from build123d import *

# Parameters (mm, degrees)
SKETCH1_R           = 23.25
BOSS_EXTRUDE1_DEPTH = 8
SKETCH2_R           = 9.6
CUT_EXTRUDE1_DEPTH  = 6.2
SKETCH3_R           = 5
CUT_EXTRUDE2_DEPTH  = 1.8
CHAMFER1_SIZE       = 2


with BuildPart() as part:
    # Sketch1 → Boss-Extrude1 (new body)
    with BuildSketch(Plane.XY):
        Circle(SKETCH1_R)
    extrude(amount=BOSS_EXTRUDE1_DEPTH)

    # Sketch2 → Cut-Extrude1 (cut)
    with BuildSketch(Plane.XY.offset(8)):
        Circle(SKETCH2_R)
    extrude(amount=-CUT_EXTRUDE1_DEPTH, mode=Mode.SUBTRACT)

    # Sketch3 → Cut-Extrude2 (cut)
    with BuildSketch(Plane.XY.offset(1.8)):
        Circle(SKETCH3_R)
    extrude(amount=-CUT_EXTRUDE2_DEPTH, mode=Mode.SUBTRACT)

    # Chamfer1
    chamfer1_edges = [part.edges().sort_by_distance(p)[0] for p in [
        (-23.25, 0, 0),
    ]]
    chamfer(chamfer1_edges, length=CHAMFER1_SIZE)


solid = part.part
The listing builds one solid part. Answer for the finished solid, in the listing's coordinates (mm). A direction names the side the tool comes from. Round coordinates to 2 decimals unless told otherwise and drop trailing zeros. Write each loop counter-clockwise with the first axis right and the second up, starting at its lowest first coordinate (ties: lowest second). Pieces come first, ordered by that corner, then holes. Notation, with made-up numbers: (67, 88) - (91, 88) arc R21 ccw to (91, 118) - close; hole circle Ø1 at (-20, 37.5). An arc over 180 degrees is marked (long way). Use a Markdown table: item, result. Add a question column.
1. Flat-ended cylindrical pins translate along their axes: P1, Ø1, axis at y = -13.5, z = 4.5, coming from the -X side; P2, Ø1.5, axis at x = -7.5, z = 4.5, coming from the -Y side; P3, Ø3, axis at y = -18, z = 3, coming from the +X side; P4, Ø9, axis at x = 0, y = 0, coming from the +Z side. Find the tip coordinate at first contact, or state that the pin passes through.
2. For a pull along X with two mould halves and no side action, classify faces 3 (the face through (22.176, 6.984, 4.958)), 4 (the face through (-1.08, -4.88, 0.91)), 5 (the face through (10, 0, 8)) as +X half, -X half, draft (parallel to the pull), parting line (faces both ways), or undercut.
3. Consider line 1 (Y direction, x = 0, z = 6.5); line 2 (X direction, y = -1, z = 3.75); line 3 (Y direction, x = 6, z = 6.75). Determine where each line is inside the solid, lowest interval first.
4. A tool of negligible diameter and unlimited length cuts with its end or side. For faces 1 (the face through (5.161, 8.095, 4.943)), 2 (the face through (4, -4, 0)), from which of +Z, -Z, +X, -X, +Y, -Y can it reach the whole face along a straight path? Write none if from no direction.
5. The part is cut by section A-A (x = 0). Write down the section's boundary in (y, z).
Reported:
| question | item | result |
|---|---|---|
| 1 | P1 | x = -19.28 |
| 1 | P2 | y = -22.25 |
| 1 | P3 | x = 16.38 |
| 1 | P4 | through |
| 2 | face 3 | parting line |
| 2 | face 4 | undercut |
| 2 | face 5 | draft |
| 3 | line 1 | -23.25 to -9.6, 9.6 to 23.25 |
| 3 | line 2 | -23.23 to -9.55, 9.55 to 23.23 |
| 3 | line 3 | -22.46 to -7.49, 7.49 to 22.46 |
| 4 | face 1 | +Z |
| 4 | face 2 | -Z, +X, -X, +Y, -Y |
| 5 | outline | (-23.25, 2) - (-21.25, 0) - (-5, 0) - (-5, 1.8) - (-9.6, 1.8) - (-9.6, 8) - (-23.25, 8) - close; (5, 0) - (21.25, 0) - (23.25, 2) - (23.25, 8) - (9.6, 8) - (9.6, 1.8) - (5, 1.8) - close |
